Answer from the drawing. Dimensions are ordinates in mm from the lowest x, y and z of the part. Give positions to 0.01 mm unless a question says otherwise; leave off trailing zeros. Order: outer loops, then holes, each group sorted by start corner. A loop starts at its lowest first (then second) coordinate and runs counter-clockwise, first axis right, second up. Notation, with made-up numbers: (5.5, 15) - (31.5, 15) arc R18 cw to (31.5, 26) - close; hole circle Ø3 at (18, 31.25). An arc over 180 degrees is marked (long way). Use a Markdown table: item, result. Add a question column.
1) Find section A-A, the plane z = 47. Determine the outline of the cut face in (x, y), plus the area to 3 significant figures.
2) Flat-ended cylindrical pins translate along their axes: pin 1 (23 mm diameter, centred on y = 16.5, z = 300.5, fed in from +X); pin 2 (2 mm diameter, centred on x = 15.5, z = 219, fed in from +Y). Find the tip coordinate at first contact, or state that the pin passes through.
3) Find section D-D, the plane z = 117. Determine the outline of the cut face in (x, y).
4) Find section C-C, the plane x = 36.5. Determine the outline of the cut face in (y, z) (1 decimal), plus the area to 3 significant figures.
5) Straight lines are drawn through the part: line 1 (Y direction, x = 12, z = 127); line 2 (X direction, y = 4.5, z = 408) (1 decimal). For each, find the intervals that lie inside material, in ascending order.
6) Find section B-B, the plane y = 35.5. Determine the outline of the cut face in (x, z) (1 decimal).
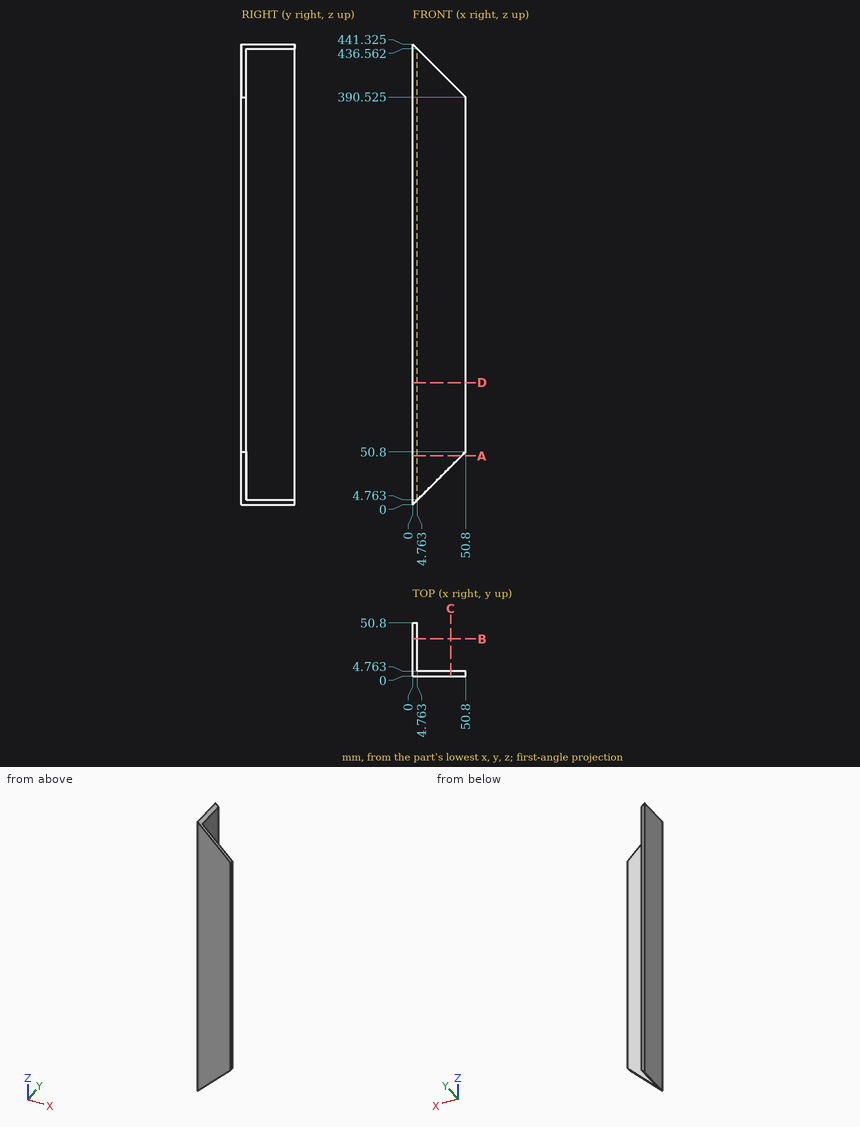
The answers:
| question | item | result |
|---|---|---|
| 1 | outline | (0, 0) - (47, 0) - (47, 4.76) - (4.76, 4.76) - (4.76, 50.8) - (0, 50.8) - close |
| 1 | area | 443 mm2 |
| 2 | pin 1 | x = 4.76 |
| 2 | pin 2 | y = 4.76 |
| 3 | outline | (0, 0) - (50.8, 0) - (50.8, 4.76) - (4.76, 4.76) - (4.76, 50.8) - (0, 50.8) - close |
| 4 | outline | (0, 36.5) - (4.8, 36.5) - (4.8, 404.8) - (0, 404.8) - close |
| 4 | area | 1,750 mm2 |
| 5 | line 1 | 0 to 4.76 |
| 5 | line 2 | 0 to 33.3 |
| 6 | outline | (0, 0) - (4.8, 4.8) - (4.8, 436.6) - (0, 441.3) - close |
